```python
from build123d import *

# Parameters (mm, degrees)
SZKIC1_R                    = 4.5
SZKIC1_R_2                  = 0.55
DODANIE_WYCI_GNI_CIE1_DEPTH = 2
SZKIC2_R                    = 0.55
WYTNIJ_WYCI_GNI_CIE1_DEPTH  = 1


with BuildPart() as part:
    # Szkic1 → Dodanie-wyciągnięcie1 (new body)
    with BuildSketch(Plane.XY):
        Circle(SZKIC1_R)
        Circle(SZKIC1_R_2, mode=Mode.SUBTRACT)
    extrude(amount=DODANIE_WYCI_GNI_CIE1_DEPTH)

    # Szkic2 → Wytnij-wyciągnięcie1 (cut)
    with BuildSketch(Plane.XY.offset(2)):
        with Locations((0, 3.25)):
            Circle(SZKIC2_R)
        with Locations((1.410122152, 2.928148821)):
            Circle(SZKIC2_R)
        with Locations((2.540952318, 2.026341856)):
            Circle(SZKIC2_R)
        with Locations((3.168515715, 0.723193035)):
            Circle(SZKIC2_R)
        with Locations((3.168515715, -0.723193035)):
            Circle(SZKIC2_R)
        with Locations((2.540952318, -2.026341856)):
            Circle(SZKIC2_R)
        with Locations((1.410122152, -2.928148821)):
            Circle(SZKIC2_R)
        with Locations((0, -3.25)):
            Circle(SZKIC2_R)
        with Locations((-1.410122152, -2.928148821)):
            Circle(SZKIC2_R)
        with Locations((-2.540952318, -2.026341856)):
            Circle(SZKIC2_R)
        with Locations((-3.168515715, -0.723193035)):
            Circle(SZKIC2_R)
        with Locations((-3.168515715, 0.723193035)):
            Circle(SZKIC2_R)
        with Locations((-2.540952318, 2.026341856)):
            Circle(SZKIC2_R)
        with Locations((-1.410122152, 2.928148821)):
            Circle(SZKIC2_R)
    extrude(amount=-WYTNIJ_WYCI_GNI_CIE1_DEPTH, mode=Mode.SUBTRACT)


solid = part.part
```
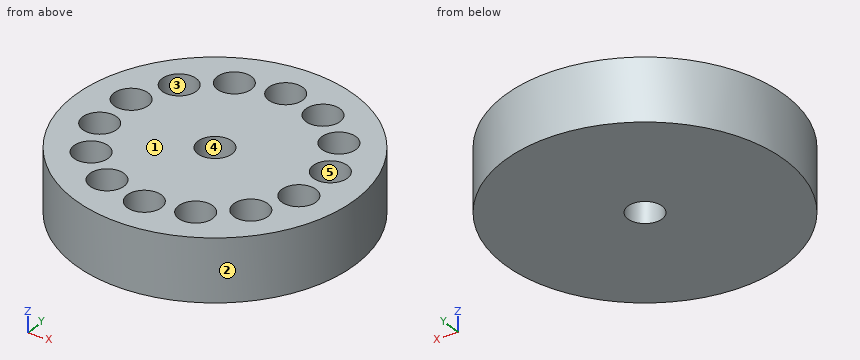
Here's how the part is built. I have some questions about the finished solid (model axes, mm). Face numbers are marked on the shaded views. A direction names the side the tool comes from. Coordinates: 2 decimals unless noted, no trailing zeros. Order: outer loops, then holes, each group sorted by start corner. A loop starts at its lowest first (then second) coordinate and runs counter-clockwise, first axis right, second up.
1) Will these pins go through, and if not, where does the flat tip stop? pin 1 (1 mm diameter, centred on x = 0, y = -3.25, fed in from +Z); pin 2 (1 mm diameter, centred on y = 1, z = 0.5, fed in from -X).
2) Imagine slicing it at D-D on x = 1.5. List the corners of the cut face in (y, z) for me.
3) Which directions (+Z, -Z, +X, -X, +Y, -Y) give clear straight access to the entire face, cutting with the end or side of a thin tool? Please do the marked faces 4 and 5.
4) Imagine slicing it at C-C on z = 0.6. List the corners of the cut face in (x, y) for me.
5) I need wall thicknesses on line 1 (Y direction, x = -1.5, z = 1.5); line 2 (Y direction, x = 1.25, z = 1.65); line 3 (Y direction, x = 0, z = 1.25). Which ranges of each line are inside material? Lowest first, please.
6) Imagine slicing it at B-B on z = 1.8. State how many separate pieces and enclosed holes the cut face has, and give its area (3 significant figures).
7) Imagine slicing it at A-A on x = 0. List the corners of the cut face in (y, z) for me, and give its area (3 significant figures).
8) We'd pull the mould along X, two halves only. Please class the marked faces 1, 2 and 3: +X half, -X half, draft (parallel to the pull), parting line (faces both ways), or undercut.
Response values:
1. pin 1: stops at z = 1
1. pin 2: stops at x = -4.47
2. outline: (-4.24, 0) - (4.24, 0) - (4.24, 2) - (3.47, 2) - (3.47, 1) - (2.39, 1) - (2.39, 2) - (-2.39, 2) - (-2.39, 1) - (-3.47, 1) - (-3.47, 2) - (-4.24, 2) - close
3. face 4: +Z, -Z
3. face 5: +Z
4. outline: circle Ø9 at (0, 0); hole circle Ø1.1 at (0, 0)
5. line 1: y = -4.24 to -3.47, -2.39 to 2.39, 3.47 to 4.24
5. line 2: y = -4.32 to -3.45, -2.4 to 2.4, 3.45 to 4.32
5. line 3: y = -4.5 to -3.8, -2.7 to -0.55, 0.55 to 2.7, 3.8 to 4.5
6. separate pieces: 1
6. enclosed holes: 15
6. area: 49.4 mm2
7. outline: (-4.5, 0) - (-0.55, 0) - (-0.55, 2) - (-2.7, 2) - (-2.7, 1) - (-3.8, 1) - (-3.8, 2) - (-4.5, 2) - close; (0.55, 0) - (4.5, 0) - (4.5, 2) - (3.8, 2) - (3.8, 1) - (2.7, 1) - (2.7, 2) - (0.55, 2) - close
7. area: 13.6 mm2
8. face 1: draft
8. face 2: parting line
8. face 3: undercut
